```python
from build123d import *

# Parameters (mm, degrees)
BOSS_EXTRUDE1_DEPTH         = 25.4
FILLET1_R                   = 12.7
F_3_4_0_75_DIAMETER_HOLE1_D = 19.05
F_1_2_0_5_DIAMETER_HOLE2_D  = 12.7


with BuildPart() as part:
    # Sketch1 → Boss-Extrude1 (new body)
    with BuildSketch(Plane.XY):
        Polygon((-38.1, 44.45), (0, 44.45), (0, 0), (50.8, 0), (50.8, 6.35), (6.35, 6.35), (6.35, 50.8), (-38.1, 50.8), align=None)
    extrude(amount=BOSS_EXTRUDE1_DEPTH)

    # Fillet1
    fillet1_edges = [part.edges().sort_by_distance(p)[0] for p in [
        (50.8, 3.175, 0),
        (-38.1, 47.625, 0),
        (50.8, 3.175, 25.4),
        (-38.1, 47.625, 25.4),
    ]]
    fillet(fillet1_edges, radius=FILLET1_R - 0.0001)  # a hair under: the kernel refuses the full size

    # 3/4 (0.75) Diameter Hole1 (through all)
    with Locations(Plane(origin=(0, 50.8, 0), x_dir=(1, 0, 0), z_dir=(0, 1, 0))):
        with Locations((-25.4, -12.7)):
            Hole(F_3_4_0_75_DIAMETER_HOLE1_D / 2)

    # 1/2 (0.5) Diameter Hole2 (through all)
    with Locations(Plane(origin=(0, 6.35, 0), x_dir=(1, 0, 0), z_dir=(0, 1, 0))):
        with Locations((38.1, -12.7)):
            Hole(F_1_2_0_5_DIAMETER_HOLE2_D / 2)


solid = part.part
```
Geometry check sheet. Reference: the model listing, model coordinates, mm. A direction names the side the tool comes from. Coordinates: 2 decimals unless noted, no trailing zeros. Loops run counter-clockwise (first coordinate to the right, second up) from the corner with the lowest first, then second, coordinate; pieces in that order, holes last. Notation, with made-up numbers: (11, -31.75) - (35, -31.75) arc R16 ccw to (35, -22.75) - close; hole circle Ø1 at (5.25, -7). An arc over 180 degrees is marked (long way). One line per item, written item: value. Start each with the question number.
(1) Cross-section at C-C on y = 29.5. Enter the section's corners in (x, z), plus the area to 3 significant figures.
(2) Mould release check, pull along X, two halves, no side actions. Record for faces 3 (the flat face through (0, 23, 13)), 4 (the cylindrical face through (32.234, 3.131, 15.132)), 5 (the cylindrical face through (47.18, 3.22, 21.58)), 6 (the flat face through (-15, 44.45, 13)): released by +X, released by -X, zero draft, split by the parting line, or undercut.
(3) Material ranges on line 1 (Z direction, x = 38.1, y = 2.75); line 2 (Z direction, x = -25, y = 46); line 3 (X direction, y = 10, z = 2.5), recorded low to high. Write a range as [from, to].
(4) Cross-section at D-D on x = -11. Enter the section's corners in (y, z).
(5) Depth check by flat-ended pin: P1, Ø6, axis at y = 39, z = 16, coming from the -X side; P2, Ø12, axis at x = 20, z = 17.5, coming from the +Y side; P3, Ø8, axis at x = 37.5, z = 10.5, coming from the -Y side; P4, Ø1.5, axis at y = 45.5, z = 11.5, coming from the +X side. Enter the tip coordinate at first touch or a pass-through.
(6) Cross-section at B-B on z = 10.5. Enter the section's corners in (x, y).
(7) Tool access check on faces 1 (the flat face through (4, 26, 0)), 2 (the flat face through (6.35, 28, 13)). Record the directions out of +Z, -Z, +X, -X, +Y, -Y that give a thin tool (end or side, any length) a straight path to the whole face; none if there is none.
(8) Cross-section at A-A on z = 5.25. Enter the section's corners in (x, y).
Results below:
1. outline: (0, 0) - (6.35, 0) - (6.35, 25.4) - (0, 25.4) - close
1. area: 161 mm2
2. face 3: released by -X
2. face 4: undercut
2. face 5: released by +X
2. face 6: zero draft
3. line 1: z = [0, 6.35], [19.05, 25.4]
3. line 2: z = [0, 3.18], [22.22, 25.4]
3. line 3: x = [0, 6.35]
4. outline: (44.45, 0) - (50.8, 0) - (50.8, 25.4) - (44.45, 25.4) - close
5. P1: stops at x = 0
5. P2: stops at y = 6.35
5. P3: passes through
5. P4: stops at x = 6.35
6. outline: (-37.91, 44.45) - (-34.67, 44.45) - (-34.67, 50.8) - (-37.91, 50.8) - close; (-16.13, 44.45) - (0, 44.45) - (0, 0) - (32.14, 0) - (32.14, 6.35) - (6.35, 6.35) - (6.35, 50.8) - (-16.13, 50.8) - close; (44.06, 0) - (50.61, 0) - (50.61, 6.35) - (44.06, 6.35) - close
7. face 1: -Z, +X, -X, +Y, -Y
7. face 2: +Z, -Z, +X, +Y
8. outline: (-35.69, 44.45) - (-31.33, 44.45) - (-31.33, 50.8) - (-35.69, 50.8) - close; (-19.47, 44.45) - (0, 44.45) - (0, 0) - (48.39, 0) - (48.39, 6.35) - (6.35, 6.35) - (6.35, 50.8) - (-19.47, 50.8) - close
